Autodesk Inventor part; units mm, degrees
sketch "Sketch1" plane through (0, 0, 0) normal (0, 0, 1) x (1, 0, 0)
  line L0 (0, 1.7864) -> (0, -1.7864) construction
  line L1 (-3.6109, 0) -> (3.6109, 0) construction
  circle A0 centre (0, 0) radius 2.5
  dimension "d0" = 5
extrude "Extrusion1" add sketch "Sketch1" along normal blind 10
sketch "Sketch2" plane through (0, 0, 10) normal (0, 0, 1) x (1, 0, 0)
  circle A0 centre (0, 0) radius 6
  dimension "d3" = 12
extrude "Extrusion2" add sketch "Sketch2" along normal blind 19
sketch "Sketch3" plane through (0, 0, 29) normal (0, 0, 1) x (1, 0, 0)
  circle A0 centre (0, 0) radius 2.5
  dimension "d6" = 5
extrude "Extrusion3" add sketch "Sketch3" along normal blind 24.5
sketch "Sketch5" plane through (0, 0, 53.5) normal (0, 0, 1) x (1, 0, 0)
  line L0 (0, 8.3226) -> (8.1221, 8.3226)
  line L1 (8.1221, 8.3226) -> (8.1221, -8.0744)
  line L2 (8.1221, -8.0744) -> (0, -8.0744)
  line L3 (0, -8.0744) -> (0, 8.3226)
  point P0 (0, 0)
extrude "Extrusion5" cut sketch "Sketch5" against normal blind 58
properties part number "Stang" material "S235"
Part model, mm, in its own coordinate system. A direction names the side the tool comes from. Give positions to 0.01 mm unless a question says otherwise; leave off trailing zeros. Order: outer loops, then holes, each group sorted by start corner. A loop starts at its lowest first (then second) coordinate and runs counter-clockwise, first axis right, second up. Notation, with made-up numbers: (-9.75, -9) - (38.25, -9) arc R27 cw to (38.25, 24) - close; hole circle Ø3 at (59, -31.75). An arc over 180 degrees is marked (long way). Use a Markdown table: item, result.
1) Probe L1, parallel to Z at x = -2.1, y = 4.75; L2, parallel to X at y = 0, z = 33; L3, parallel to X at y = -0.5, z = 22. List the from-to ranges inside material, lowest first. Write a range as from..to.
Checked values:
| item | result |
|---|---|
| L1 | 10..29 |
| L2 | -2.5..0 |
| L3 | -5.98..0 |
2) Saw through at D-D on x = -4.7. List the corners of the cut face in (y, z), plus the area to 3 significant figures.
Checked values:
| item | result |
|---|---|
| outline | (-3.73, 10) - (3.73, 10) - (3.73, 29) - (-3.73, 29) - close |
| area | 142 mm² |
3) Saw through at A-A on y = 0. List the corners of the cut face in (x, z), plus the area to 3 significant figures.
Checked values:
| item | result |
|---|---|
| outline | (-6, 10) - (-2.5, 10) - (-2.5, 0) - (0, 0) - (0, 53.5) - (-2.5, 53.5) - (-2.5, 29) - (-6, 29) - close |
| area | 200 mm² |
4) Saw through at B-B on x = -0.9. List the corners of the cut face in (y, z), plus the area to 3 significant figures.
Checked values:
| item | result |
|---|---|
| outline | (-5.93, 10) - (-2.33, 10) - (-2.33, 0) - (2.33, 0) - (2.33, 10) - (5.93, 10) - (5.93, 29) - (2.33, 29) - (2.33, 53.5) - (-2.33, 53.5) - (-2.33, 29) - (-5.93, 29) - close |
| area | 386 mm² |
5) Flat gauge pins, fed straight in: P1, Ø4, axis at y = 0, z = 8.5, coming from the +X side; P2, Ø1.8, axis at x = -3.5, y = 0, coming from the -Z side; P3, Ø2, axis at x = -4, z = 29, coming from the -Y side; P4, Ø1, axis at x = -2.5, y = 4.5, coming from the +Z side. Where does each tip first touch, or does it go through?
Checked values:
| item | result |
|---|---|
| P1 | x = 0 |
| P2 | z = 10 |
| P3 | y = -5.2 |
| P4 | z = 29 |
6) 3-axis set-ups, long thin cutter, end or side, ignore diameter. For faces 1 (the cylindrical face through (-2.5, -0.1, 4.9)), 2 (the flat face through (0, 0, 27)), 3 (the cylindrical face through (-2.5, -0.1, 41.1)): which of +Z, -Z, +X, -X, +Y, -Y reach the whole face in a straight line?
Checked values:
| item | result |
|---|---|
| face 1 | -Z, -X |
| face 2 | +Z, -Z, +X, +Y, -Y |
| face 3 | +Z, -X |
7) Saw through at C-C on z = 43.5. List the corners of the cut face in (x, y), plus the area to 3 significant figures.
Checked values:
| item | result |
|---|---|
| outline | (0, -2.5) - (0, 2.5) arc R2.5 ccw to start |
| area | 9.82 mm² |
